Work out the finished part from the listing and answer in its coordinate system (mm). Face numbers are marked on the shaded views. Round coordinates to 2 decimals unless told otherwise and drop trailing zeros. Write each loop counter-clockwise with the first axis right and the second up, starting at its lowest first coordinate (ties: lowest second). Pieces come first, ordered by that corner, then holes. Notation, with made-up numbers: M -26,47 L 11,47 A13 ccw 11,59 Z; hole C -18,-30.75 d9. An arc over 180 degrees is marked long. One line per item, written item: value. Start each with the question number.
Q1. Consider probe 1 along X at (y, z) = (3.75, 0); probe 2 along X at (y, z) = (3.5, -1); probe 3 along Z at (x, y) = (-0.5, 1). Determine where each line is inside the solid, lowest interval first.
Q2. Find section A-A (y = 1.5). Count the separate pieces of the cut face and the enclosed holes in it, and give its area (3 significant figures).
Q3. Find section B-B (z = -12.5). Write down the section's boundary in (x, y), and give its area (3 significant figures).
Q4. The mould has two halves that part along X. Classify the marked faces 1, 2 and 3: released by +X, released by -X, zero draft, split by the parting line, or undercut.
Q5. Given pin 1 Ø2.5 at (x, z) = (7.5, 0) entering from +Y; pin 2 Ø3 at (x, y) = (-4, 8) entering from -Z; pin 3 Ø5 at (y, z) = (7.5, 5) entering from -X; pin 4 Ø3 at (y, z) = (5, -1.5) entering from -X, each flat-ended and moving along its own axis, determine where each tip first touches the part or whether it passes through.
from build123d import *

# Parameters (mm, degrees)
BOSS_EXTRUDE1_DEPTH = 8
SKETCH2_R           = 15
BOSS_EXTRUDE2_DEPTH = 1.5
SKETCH4_R           = 2.5
CUT_EXTRUDE1_DEPTH  = 23
SKETCH5_R           = 1.5
CUT_EXTRUDE2_DEPTH  = 24.243278598


with BuildPart() as part:
    # Sketch1 → Boss-Extrude1 (new body)
    with BuildSketch(Plane(origin=(0, 0, 0), x_dir=(1, 0, 0), z_dir=(0, 1, 0))):
        with BuildLine():
            ThreePointArc((-2.619011045, 11.679969227), (-2.794341005, 11.639267947), (-2.969039138, 11.595934917))
            ThreePointArc((-2.969039138, 11.595934917), (-3.464080507, 10.661343548), (-4.413916411, 11.126465832))
            ThreePointArc((-4.413916411, 11.126465832), (-4.580720685, 11.058838004), (-4.746489215, 10.988709666))
            ThreePointArc((-4.746489215, 10.988709666), (-5.089233502, 9.988183136), (-6.100136506, 10.298991922))
            ThreePointArc((-6.100136506, 10.298991922), (-6.25430782, 10.206102767), (-6.407064974, 10.110905915))
            ThreePointArc((-6.407064974, 10.110905915), (-6.589072678, 9.069080507), (-7.636150994, 9.21792265))
            ThreePointArc((-7.636150994, 9.21792265), (-7.773893139, 9.102059408), (-7.909877531, 8.984138103))
            ThreePointArc((-7.909877531, 8.984138103), (-7.926667017, 7.926667017), (-8.984138103, 7.909877531))
            ThreePointArc((-8.984138103, 7.909877531), (-9.102059408, 7.773893139), (-9.21792265, 7.636150994))
            ThreePointArc((-9.21792265, 7.636150994), (-9.069080507, 6.589072678), (-10.110905915, 6.407064974))
            ThreePointArc((-10.110905915, 6.407064974), (-10.206102767, 6.25430782), (-10.298991922, 6.100136506))
            ThreePointArc((-10.298991922, 6.100136506), (-9.988183136, 5.089233502), (-10.988709666, 4.746489215))
            ThreePointArc((-10.988709666, 4.746489215), (-11.058838004, 4.580720685), (-11.126465832, 4.413916411))
            ThreePointArc((-11.126465832, 4.413916411), (-10.661343548, 3.464080507), (-11.595934917, 2.969039138))
            ThreePointArc((-11.595934917, 2.969039138), (-11.639267947, 2.794341005), (-11.679969227, 2.619011045))
            ThreePointArc((-11.679969227, 2.619011045), (-11.071986298, 1.753630353), (-11.917629765, 1.118481464))
            ThreePointArc((-11.917629765, 1.118481464), (-11.933100485, 0.939155376), (-11.945873016, 0.759616935))
            ThreePointArc((-11.945873016, 0.759616935), (-11.21, 0), (-11.945873016, -0.759616935))
            ThreePointArc((-11.945873016, -0.759616935), (-11.933100485, -0.939155376), (-11.917629765, -1.118481464))
            ThreePointArc((-11.917629765, -1.118481464), (-11.071986298, -1.753630353), (-11.679969227, -2.619011045))
            ThreePointArc((-11.679969227, -2.619011045), (-11.639267947, -2.794341005), (-11.595934917, -2.969039138))
            ThreePointArc((-11.595934917, -2.969039138), (-10.661343548, -3.464080507), (-11.126465832, -4.413916411))
            ThreePointArc((-11.126465832, -4.413916411), (-11.058838004, -4.580720685), (-10.988709666, -4.746489215))
            ThreePointArc((-10.988709666, -4.746489215), (-9.988183136, -5.089233502), (-10.298991922, -6.100136506))
            ThreePointArc((-10.298991922, -6.100136506), (-10.206102767, -6.25430782), (-10.110905915, -6.407064974))
            ThreePointArc((-10.110905915, -6.407064974), (-9.069080507, -6.589072678), (-9.21792265, -7.636150994))
            ThreePointArc((-9.21792265, -7.636150994), (-9.102059408, -7.773893139), (-8.984138103, -7.909877531))
            ThreePointArc((-8.984138103, -7.909877531), (-7.926667017, -7.926667017), (-7.909877531, -8.984138103))
            ThreePointArc((-7.909877531, -8.984138103), (-7.773893139, -9.102059408), (-7.636150994, -9.21792265))
            ThreePointArc((-7.636150994, -9.21792265), (-6.589072678, -9.069080507), (-6.407064974, -10.110905915))
            ThreePointArc((-6.407064974, -10.110905915), (-6.25430782, -10.206102767), (-6.100136506, -10.298991922))
            ThreePointArc((-6.100136506, -10.298991922), (-5.089233502, -9.988183136), (-4.746489215, -10.988709666))
            ThreePointArc((-4.746489215, -10.988709666), (-4.580720685, -11.058838004), (-4.413916411, -11.126465832))
            ThreePointArc((-4.413916411, -11.126465832), (-3.464080507, -10.661343548), (-2.969039138, -11.595934917))
            ThreePointArc((-2.969039138, -11.595934917), (-2.794341005, -11.639267947), (-2.619011045, -11.679969227))
            ThreePointArc((-2.619011045, -11.679969227), (-1.753630353, -11.071986298), (-1.118481464, -11.917629765))
            ThreePointArc((-1.118481464, -11.917629765), (-0.939155376, -11.933100485), (-0.759616935, -11.945873016))
            ThreePointArc((-0.759616935, -11.945873016), (0, -11.21), (0.759616935, -11.945873016))
            ThreePointArc((0.759616935, -11.945873016), (0.939155376, -11.933100485), (1.118481464, -11.917629765))
            ThreePointArc((1.118481464, -11.917629765), (1.753630353, -11.071986298), (2.619011045, -11.679969227))
            ThreePointArc((2.619011045, -11.679969227), (2.794341005, -11.639267947), (2.969039138, -11.595934917))
            ThreePointArc((2.969039138, -11.595934917), (3.464080507, -10.661343548), (4.413916411, -11.126465832))
            ThreePointArc((4.413916411, -11.126465832), (4.580720685, -11.058838004), (4.746489215, -10.988709666))
            ThreePointArc((4.746489215, -10.988709666), (5.089233502, -9.988183136), (6.100136506, -10.298991922))
            ThreePointArc((6.100136506, -10.298991922), (6.25430782, -10.206102767), (6.407064974, -10.110905915))
            ThreePointArc((6.407064974, -10.110905915), (6.589072678, -9.069080507), (7.636150994, -9.21792265))
            ThreePointArc((7.636150994, -9.21792265), (7.773893139, -9.102059408), (7.909877531, -8.984138103))
            ThreePointArc((7.909877531, -8.984138103), (7.926667017, -7.926667017), (8.984138103, -7.909877531))
            ThreePointArc((8.984138103, -7.909877531), (9.102059408, -7.773893139), (9.21792265, -7.636150994))
            ThreePointArc((9.21792265, -7.636150994), (9.069080507, -6.589072678), (10.110905915, -6.407064974))
            ThreePointArc((10.110905915, -6.407064974), (10.206102767, -6.25430782), (10.298991922, -6.100136506))
            ThreePointArc((10.298991922, -6.100136506), (9.988183136, -5.089233502), (10.988709666, -4.746489215))
            ThreePointArc((10.988709666, -4.746489215), (11.058838004, -4.580720685), (11.126465832, -4.413916411))
            ThreePointArc((11.126465832, -4.413916411), (10.661343548, -3.464080507), (11.595934917, -2.969039138))
            ThreePointArc((11.595934917, -2.969039138), (11.639267947, -2.794341005), (11.679969227, -2.619011045))
            ThreePointArc((11.679969227, -2.619011045), (11.071986298, -1.753630353), (11.917629765, -1.118481464))
            ThreePointArc((11.917629765, -1.118481464), (11.933100485, -0.939155376), (11.945873016, -0.759616935))
            ThreePointArc((11.945873016, -0.759616935), (11.21, 0), (11.945873016, 0.759616935))
            ThreePointArc((11.945873016, 0.759616935), (11.933100485, 0.939155376), (11.917629765, 1.118481464))
            ThreePointArc((11.917629765, 1.118481464), (11.071986298, 1.753630353), (11.679969227, 2.619011045))
            ThreePointArc((11.679969227, 2.619011045), (11.639267947, 2.794341005), (11.595934917, 2.969039138))
            ThreePointArc((11.595934917, 2.969039138), (10.661343548, 3.464080507), (11.126465832, 4.413916411))
            ThreePointArc((11.126465832, 4.413916411), (11.058838004, 4.580720685), (10.988709666, 4.746489215))
            ThreePointArc((10.988709666, 4.746489215), (9.988183136, 5.089233502), (10.298991922, 6.100136506))
            ThreePointArc((10.298991922, 6.100136506), (10.206102767, 6.25430782), (10.110905915, 6.407064974))
            ThreePointArc((10.110905915, 6.407064974), (9.069080507, 6.589072678), (9.21792265, 7.636150994))
            ThreePointArc((9.21792265, 7.636150994), (9.102059408, 7.773893139), (8.984138103, 7.909877531))
            ThreePointArc((8.984138103, 7.909877531), (7.926667017, 7.926667017), (7.909877531, 8.984138103))
            ThreePointArc((7.909877531, 8.984138103), (7.773893139, 9.102059408), (7.636150994, 9.21792265))
            ThreePointArc((7.636150994, 9.21792265), (6.589072678, 9.069080507), (6.407064974, 10.110905915))
            ThreePointArc((6.407064974, 10.110905915), (6.25430782, 10.206102767), (6.100136506, 10.298991922))
            ThreePointArc((6.100136506, 10.298991922), (5.089233502, 9.988183136), (4.746489215, 10.988709666))
            ThreePointArc((4.746489215, 10.988709666), (4.580720685, 11.058838004), (4.413916411, 11.126465832))
            ThreePointArc((4.413916411, 11.126465832), (3.464080507, 10.661343548), (2.969039138, 11.595934917))
            ThreePointArc((2.969039138, 11.595934917), (2.794341005, 11.639267947), (2.619011045, 11.679969227))
            ThreePointArc((2.619011045, 11.679969227), (1.753630353, 11.071986298), (1.118481464, 11.917629765))
            ThreePointArc((1.118481464, 11.917629765), (0.939155376, 11.933100485), (0.759616935, 11.945873016))
            ThreePointArc((0.759616935, 11.945873016), (0, 11.21), (-0.759616935, 11.945873016))
            ThreePointArc((-0.759616935, 11.945873016), (-0.939155376, 11.933100485), (-1.118481464, 11.917629765))
            ThreePointArc((-1.118481464, 11.917629765), (-1.753630353, 11.071986298), (-2.619011045, 11.679969227))
        make_face()
    extrude(amount=BOSS_EXTRUDE1_DEPTH)

    # Sketch2 → Boss-Extrude2 (add)
    with BuildSketch(Plane(origin=(0, 8, 0), x_dir=(1, 0, 0), z_dir=(0, 1, 0))):
        with Locations(Location((0, 0, 0), (0, 0, 270))):
            Circle(SKETCH2_R)
    extrude(amount=BOSS_EXTRUDE2_DEPTH)

    # Sketch4 → Cut-Extrude1 (cut)
    with BuildSketch(Plane.XZ):
        with Locations(Location((0, 0, 0), (0, 0, 270))):
            Circle(SKETCH4_R)
    extrude(amount=-CUT_EXTRUDE1_DEPTH, mode=Mode.SUBTRACT)

    # Sketch5 → Cut-Extrude2 (cut, through all)
    with BuildSketch(Plane.XZ):
        with Locations(Location((0, 7.5, 0), (0, 0, 270))):
            Circle(SKETCH5_R)
        with Locations(Location((7.5, 0, 0), (0, 0, 270))):
            Circle(SKETCH5_R)
        with Locations(Location((0, -7.5, 0), (0, 0, 270))):
            Circle(SKETCH5_R)
        with Locations(Location((-7.5, 0, 0), (0, 0, 270))):
            Circle(SKETCH5_R)
    extrude(amount=-CUT_EXTRUDE2_DEPTH, mode=Mode.SUBTRACT)


solid = part.part
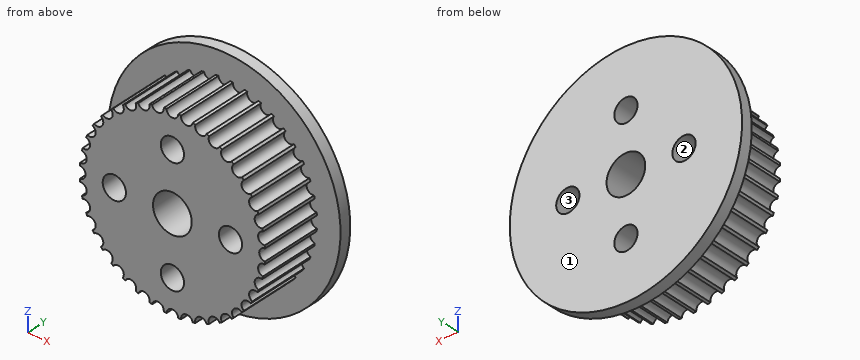
The answers:
1. probe 1: -11.21 to -9, -6 to -2.5, 2.5 to 6, 9 to 11.21
1. probe 2: -11.93 to -8.62, -6.38 to -2.29, 2.29 to 6.38, 8.62 to 11.93
1. probe 3: -11.4 to -8.91, -6.09 to -2.45, 2.45 to 6.09, 8.91 to 11.4
2. separate pieces: 1
2. enclosed holes: 5
2. area: 366 mm2
3. outline: M -8.29,8 L 8.29,8 L 8.29,9.5 L -8.29,9.5 Z
3. area: 24.9 mm2
4. face 1: zero draft
4. face 2: undercut
4. face 3: undercut
5. pin 1: through
5. pin 2: z = -14.79
5. pin 3: x = -14.78
5. pin 4: x = -11.95
